Source: CAD feature listing. Evaluate the final solid. Frame: model axes, mm. A direction names the side the tool comes from. Coordinates: 2 decimals unless noted, no trailing zeros. Order: outer loops, then holes, each group sorted by start corner. A loop starts at its lowest first (then second) coordinate and runs counter-clockwise, first axis right, second up.
```python
from build123d import *

# Parameters (mm, degrees)
F1_DEPTH = 42
F2_R     = 9
F2_R_2   = 1.5
F3_DEPTH = 30.001
F4_R     = 1.6
F5_DEPTH = 30.001


with BuildPart() as f1:
    # F0 (on Front) → F1 (new body)
    with BuildSketch(Plane.XZ):
        Polygon((0, 0), (0, 30), (-3, 30), (-3, 3), (-30, 3), (-30, 0), align=None)
    extrude(amount=F1_DEPTH)

    # F2 (on face) → F3 (cut, through all)
    with BuildSketch(Plane.YZ):
        with Locations((-21, 15)):
            Circle(F2_R)
        with Locations((-3.5, 15)):
            Circle(F2_R_2)
        with Locations((-38.5, 15)):
            Circle(F2_R_2)
    extrude(amount=-F3_DEPTH, mode=Mode.SUBTRACT)

    # F4 (on face) → F5 (cut, through all)
    with BuildSketch(Plane(origin=(0, 0, 0), x_dir=(1, 0, 0), z_dir=(0, 0, -1))):
        with Locations((-15, 11)):
            Circle(F4_R)
        with Locations((-15, 31)):
            Circle(F4_R)
    extrude(amount=-F5_DEPTH, mode=Mode.SUBTRACT)


solid = f1.part
```
1. Section query C-C on x = -15. Return loops of the section in (y, z).
Findings:
outline: (-42, 0) - (-32.6, 0) - (-32.6, 3) - (-42, 3) - close; (-29.4, 0) - (-12.6, 0) - (-12.6, 3) - (-29.4, 3) - close; (-9.4, 0) - (0, 0) - (0, 3) - (-9.4, 3) - close
2. Access query for faces 4 (the face through (-16, -21, 3)), 5 (the face through (-30, -21, 2)). Directions: +Z, -Z, +X, -X, +Y, -Y. A direction counts if a zero-diameter tool reaches every point of the face in a straight line with its end or side. Return the directions, or none.
Findings:
face 4: +Z, -X, +Y, -Y
face 5: +Z, -Z, -X, +Y, -Y
3. Draft query along Z for faces 1 (the face through (-15, -21, 0)), 2 (the face through (-1.479, -2.114, 14.425)), 3 (the face through (-8.4, 0, 2.8)). Return one class per face: released by +Z, released by -Z, zero draft, split by the parting line, or undercut.
Findings:
face 1: released by -Z
face 2: undercut
face 3: zero draft
4. Section query B-B on z = 15. Return loops of the section in (x, y).
Findings:
outline: (-3, -42) - (0, -42) - (0, -40) - (-3, -40) - close; (-3, -37) - (0, -37) - (0, -30) - (-3, -30) - close; (-3, -12) - (0, -12) - (0, -5) - (-3, -5) - close; (-3, -2) - (0, -2) - (0, 0) - (-3, 0) - close
5. Section query D-D on z = 21.75. Return loops of the section in (x, y).
Findings:
outline: (-3, -42) - (0, -42) - (0, -26.95) - (-3, -26.95) - close; (-3, -15.05) - (0, -15.05) - (0, 0) - (-3, 0) - close
6. Ray query, line 1 (Y direction, x = -15, z = 1.5); line 2 (X direction, y = -31, z = 0.75); line 3 (Z direction, x = -1.35, y = -21). Return the intervals inside material, ascending.
Findings:
line 1: y = -42 to -32.6, -29.4 to -12.6, -9.4 to 0
line 2: x = -30 to -16.6, -13.4 to 0
line 3: z = 0 to 6, 24 to 30
7. Pin query (flat end, axial travel): P1, Ø4, axis at y = -9, z = 22.5, coming from the -X side; P2, Ø4, axis at x = -15, y = -11, coming from the +Z side; P3, Ø11, axis at y = -21, z = 15, coming from the -X side. Return the tip coordinate at first contact, or that it passes through.
Findings:
P1: stops at x = -3
P2: stops at z = 3
P3: passes through
8. Section query A-A on y = -31. Return loops of the section in (x, z), plus the area to 3 significant figures.
Findings:
outline: (-30, 0) - (-16.6, 0) - (-16.6, 3) - (-30, 3) - close; (-13.4, 0) - (0, 0) - (0, 30) - (-3, 30) - (-3, 3) - (-13.4, 3) - close
area: 161 mm2
